The drawing under review shows one solid part. Ordinate dimensions are in mm from its lowest x, y, z. A direction names the side the tool comes from. Coordinates: 2 decimals unless noted, no trailing zeros. Write each loop counter-clockwise with the first axis right and the second up, starting at its lowest first coordinate (ties: lowest second). Pieces come first, ordered by that corner, then holes. Notation, with made-up numbers: (28, -3.5) -> (49, -3.5) arc R22 ccw to (49, 22.5) -> close; hole circle Ø8 at (47.25, 5). An arc over 180 degrees is marked (long way). One line per question, with ' | ' between items. Start each with the question number.
Q1. Draft analysis for pull direction X (two halves, no side actions). For the marked faces 1, 2 and 3, state which applies: pulls with the +X half, pulls with the -X half, needs draft (parallel to the pull), parting line crosses it, or undercut.
Q2. For the marked faces 4 and 5, list the 3-axis set-ups (+Z, -Z, +X, -X, +Y, -Y) from which the entire face can be reached by the end or side of a thin tool; tool diameter is ignored.
Q3. Wall thickness on probe 1 along Y at (x, z) = (12.5, 1.1); probe 2 along Y at (x, z) = (12.5, 11); probe 3 along Z at (x, y) = (13.5, 18.75): over which ranges is each line inside the solid? List them lowest first.
Q4. For P1, Ø4, axis at x = 9, y = 12, coming from the -Z side; P2, Ø10, axis at x = 6, z = 5.5, coming from the +Y side; P3, Ø10, axis at y = 3, z = 27.5, coming from the +X side; P4, Ø3, axis at x = 12.5, y = 12.5, coming from the +Z side, all flat-tipped, find the tip position at first contact; note any pin that passes through.
Q5. Add section C-C on z = 33.5. State the section outline as (x, y) points.
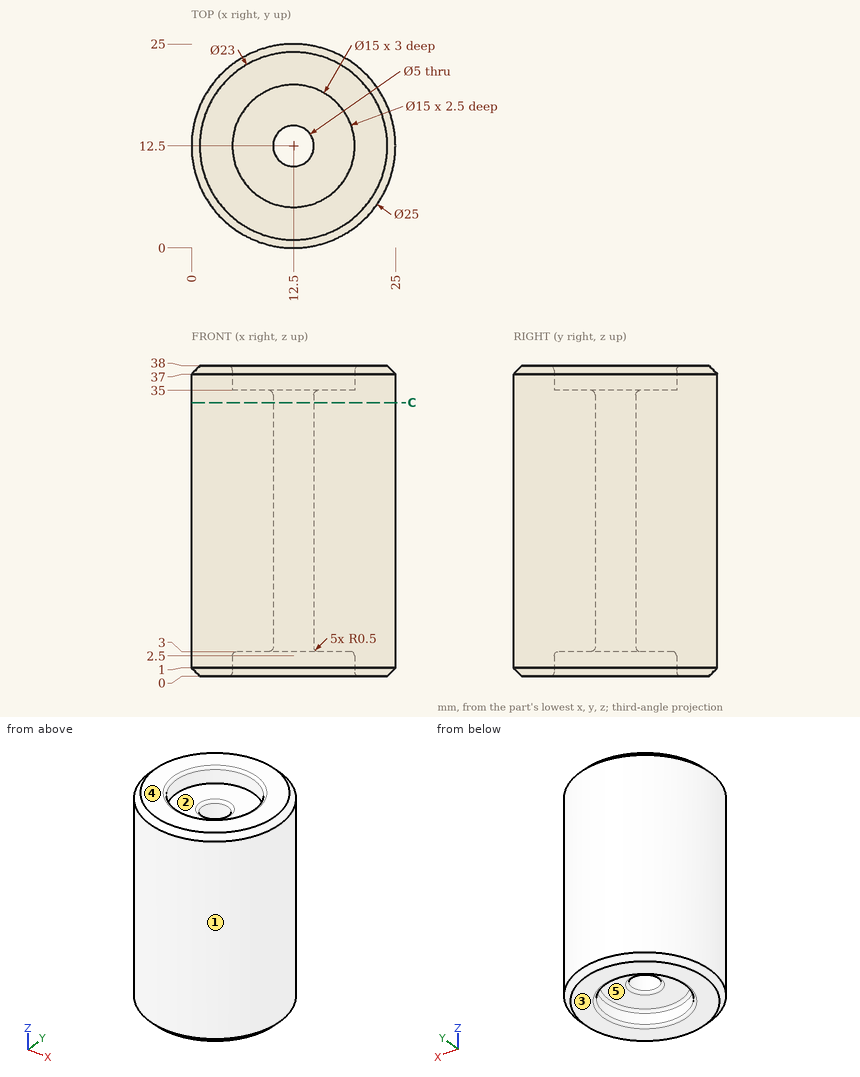
Output values:
1) face 1: parting line crosses it | face 2: undercut | face 3: needs draft
2) face 4: +Z, +X, -X, +Y, -Y | face 5: -Z
3) probe 1: y = 0 to 5, 20 to 25 | probe 2: y = 0 to 10, 15 to 25 | probe 3: z = 3 to 35
4) P1: stops at z = 3 | P2: stops at y = 24.91 | P3: stops at x = 24.16 | P4: passes through
5) outline: circle Ø25 at (12.5, 12.5); hole circle Ø5 at (12.5, 12.5)
